from build123d import *

# Parameters (mm, degrees)
BOSS_EXTRUDE1_DEPTH = 500
SKETCH2_W           = 750
SKETCH2_H           = 950
CUT_EXTRUDE1_DEPTH  = 480
SKETCH3_W           = 750
SKETCH3_H           = 950
BOSS_EXTRUDE2_DEPTH = 10


with BuildPart() as part:
    # Sketch1 → Boss-Extrude1 (new, symmetric)
    with BuildSketch(Plane.XY):
        Polygon((-500, 0), (500, 0), (500, 500), (-300, 500), (-500, 300), align=None)
    extrude(amount=BOSS_EXTRUDE1_DEPTH, both=True)

    # Sketch2 → Cut-Extrude1 (cut)
    with BuildSketch(Plane(origin=(0, 500, 0), x_dir=(1, 0, 0), z_dir=(0, 1, 0))):
        with Locations((100, 0)):
            Rectangle(SKETCH2_W, SKETCH2_H)
    extrude(amount=-CUT_EXTRUDE1_DEPTH, mode=Mode.SUBTRACT)

    # Sketch3 → Boss-Extrude2 (add)
    with BuildSketch(Plane(origin=(0, 500, 0), x_dir=(1, 0, 0), z_dir=(0, 1, 0))):
        with Locations((100, 0)):
            Rectangle(SKETCH3_W, SKETCH3_H)
    extrude(amount=-BOSS_EXTRUDE2_DEPTH)


solid = part.part
Source: CAD feature listing. Evaluate the final solid. Frame: model axes, mm. A direction names the side the tool comes from. Coordinates: 2 decimals unless noted, no trailing zeros. Loops run counter-clockwise (first coordinate to the right, second up) from the corner with the lowest first, then second, coordinate; pieces in that order, holes last. Notation, with made-up numbers: (12, 60.25) - (54, 60.25) arc R19 cw to (54, 71.25) - close; hole circle Ø8 at (-16.75, -10.5). An arc over 180 degrees is marked (long way). One line per question, with ' | ' between items.
1) Set-up query: faces 4 (the face through (-7, 0, 7)), 5 (the face through (95, 258, -475)). Return all of +Z, -Z, +X, -X, +Y, -Y with unobstructed straight access to the full face (end or side cutting, diameter ignored); none if empty.
Report:
face 4: +Z, -Z, +X, -X, -Y | face 5: none
2) Line query: line 1 along Z through (x, y) = (146, 403); line 2 along X through (y, z) = (104, 410.5); line 3 along Y through (x, z) = (-48.5, 361). Output: solid intervals per line, ascending.
Report:
line 1: z = -500 to -475, 475 to 500 | line 2: x = -500 to -275, 475 to 500 | line 3: y = 0 to 20, 490 to 500
3) First-contact query: P1, Ø1.5, axis at x = -288.5, z = -179, coming from the -Y side. Flat tip, straight axial feed; report the tip coordinate or a pass-through.
Report:
P1: stops at y = 0
4) Pull-direction query (Y, two-part tool) for faces 1 (the face through (95, 20, -7)), 2 (the face through (-7, 254, 500)), 3 (the face through (-399, 401, 7)); classes: released by +Y, released by -Y, zero draft, split by the parting line, or undercut.
Report:
face 1: undercut | face 2: zero draft | face 3: released by +Y
5) Section D-D, the plane x = -348. Return loops of the section in (y, z), then the cut area to 3 significant figures.
Report:
outline: (0, -500) - (452, -500) - (452, 500) - (0, 500) - close | area: 452,000 mm²
6) Section C-C, the plane z = 390. Return loops of the section in (x, y), then the cut area to 4 significant figures.
Report:
outline: (-500, 0) - (500, 0) - (500, 500) - (-300, 500) - (-500, 300) - close; hole (-275, 20) - (475, 20) - (475, 490) - (-275, 490) - close | area: 127,500 mm²
7) Section B-B, the plane x = -109.5. Return loops of the section in (y, z).
Report:
outline: (0, -500) - (500, -500) - (500, 500) - (0, 500) - close; hole (20, -475) - (490, -475) - (490, 475) - (20, 475) - close
8) Section A-A, the plane y = 324. Return loops of the section in (x, z).
Report:
outline: (-476, -500) - (500, -500) - (500, 500) - (-476, 500) - close; hole (-275, -475) - (475, -475) - (475, 475) - (-275, 475) - close
